For this review, take the finished solid that the model builds, in its own axes (mm). A direction names the side the tool comes from. Give positions to 0.01 mm unless a question says otherwise; leave off trailing zeros. Order: outer loops, then holes, each group sorted by start corner. A loop starts at its lowest first (then second) coordinate and runs counter-clockwise, first axis right, second up. Notation, with made-up numbers: (70, 63.5) - (110, 63.5) arc R10 ccw to (110, 76.5) - close; hole circle Ø7 at (-2, 32). An arc over 180 degrees is marked (long way). Answer as a JSON object with one key per item and string values. Group by question number.
Autodesk Inventor part; units mm, degrees
ref_plane "YZ Plane" through (0, 0, 0) normal (1, 0, 0) x (0, 1, 0)
ref_plane "XZ Plane" through (0, 0, 0) normal (0, 1, 0) x (-1, 0, 0)
ref_plane "XY Plane" through (0, 0, 0) normal (0, 0, 1) x (1, 0, 0)
sketch "Sketch1" plane through (0, 0, 0) normal (0, 0, 1) x (1, 0, 0)
  circle A0 centre (0, 0) radius 14.31
  line L0 (-76.3322, -50.4809) -> (-44.9013, -19.05)
  line L1 (0, -91.3278) -> (0, 37.4463)
  line L2 (0, -19.05) -> (-53.8815, -72.9315)
  line L3 (-53.8815, -72.9315) -> (-76.3322, -50.4809)
  line L4 (0, 19.05) -> (-105.5841, 19.05)
  line L5 (-105.5841, 19.05) -> (-159.4656, -34.8315)
  line L6 (-159.4656, -34.8315) -> (-137.015, -57.2822)
  line L7 (-137.015, -57.2822) -> (-98.7828, -19.05)
  line L8 (-98.7828, -19.05) -> (-44.9013, -19.05)
  line L9 (76.3322, -50.4809) -> (44.9013, -19.05)
  line L10 (0, -19.05) -> (53.8815, -72.9315)
  line L11 (53.8815, -72.9315) -> (76.3322, -50.4809)
  line L12 (0, 19.05) -> (105.5841, 19.05)
  line L13 (105.5841, 19.05) -> (159.4656, -34.8315)
  line L14 (159.4656, -34.8315) -> (137.015, -57.2822)
  line L15 (137.015, -57.2822) -> (98.7828, -19.05)
  line L16 (98.7828, -19.05) -> (44.9013, -19.05)
  line L17 (0, -19.05) -> (-10.6721, -29.7221)
  point P0 (-66.8959, -41.0446)
  dimension "d1" = 28.62
  dimension "d4" = 76.2
  dimension "d6" = 45
  dimension "d15" = 31.75
  dimension "d59" = 31.75
  dimension "d61" = 101.6
  dimension "d62" = 38.1
  dimension "d63" = 19.05
  dimension "d83" = 19.05
extrude "Extrusion1" add sketch "Sketch1" along normal blind 3.175 contours A0 L1 L12 L13 L14 L15 L16 L9 L11 L10 | A0 L1 L2 L3 L0 L8 L7 L6 L5 L4
sketch "Sketch3" plane through (0, 0, 3.175) normal (0, 0, 1) x (1, 0, 0)
  line L0 (53.8815, -72.9315) -> (76.3322, -50.4809)
  line L1 (76.3322, -50.4809) -> (44.9013, -19.05)
  line L2 (44.9013, -19.05) -> (98.7828, -19.05)
  line L3 (98.7828, -19.05) -> (137.015, -57.2822)
  line L4 (137.015, -57.2822) -> (159.4656, -34.8315)
  line L5 (159.4656, -34.8315) -> (105.5841, 19.05)
  line L6 (105.5841, 19.05) -> (-105.5841, 19.05)
  line L7 (-105.5841, 19.05) -> (-159.4656, -34.8315)
  line L8 (-159.4656, -34.8315) -> (-137.015, -57.2822)
  line L9 (-137.015, -57.2822) -> (-98.7828, -19.05)
  line L10 (-98.7828, -19.05) -> (-44.9013, -19.05)
  line L11 (-44.9013, -19.05) -> (-76.3322, -50.4809)
  line L12 (-76.3322, -50.4809) -> (-53.8815, -72.9315)
  line L13 (-53.8815, -72.9315) -> (0, -19.05)
  line L14 (0, -19.05) -> (53.8815, -72.9315)
  circle A0 centre (0, 0) radius 14.31
  line L15 (-148.2403, -46.0569) -> (-83.1335, 19.05)
  line L16 (-65.1069, -61.7062) -> (15.6494, 19.05)
  circle A1 centre (-139.2601, -37.0766) radius 2.65
  circle A2 centre (-121.2995, -19.1161) radius 2.65
  circle A3 centre (-103.339, -1.1556) radius 2.65
  circle A4 centre (-56.1266, -52.726) radius 2.65
  circle A5 centre (-38.1661, -34.7654) radius 2.65
  circle A6 centre (-20.2056, -16.8049) radius 2.65
  dimension "d64" = 5.3
  dimension "d67" = 25.4
  dimension "d72" = 12.7
  dimension "d73" = 12.7
  dimension "d76" = 25.4
extrude "Extrusion3" cut sketch "Sketch3" against normal blind 25.4 contours A4 L16 | L16 A4 | A5 L16 | L16 A5 | A6 L16 | L16 A6 | A3 L15 | L15 A3 | A1 L15 | L15 A1 | A2 L15 | L15 A2
mirror "Mirror2" about plane through (0, 0, 0) normal (1, 0, 0) of "Extrusion3"
fillet "Fillet1" radius 12.7 3 edges at (-98.7828, -19.05, 1.5875) (0, -19.05, 1.5875) (98.7828, -19.05, 1.5875)
fillet "Fillet2" radius 3.175 2 edges at (-44.9013, -19.05, 1.5875) (44.9013, -19.05, 1.5875)
equation "\"d1\" = bearingDiameter"
equation "\"d4\" = boltedLength"
equation "\"d6\" = 0.5 * theta12"
equation "\"d59\" = d15"
equation "\"d61\" = gearboxLength"
equation "\"topDiameter\" = 45"
equation "\"bearingDiameter\" = 28.62"
equation "\"plateThickness\" = 6.35"
equation "\"theta12\" = 90deg"
equation "\"gearboxLength\" = 101.6"
equation "\"boltedLength\" = 76.2"
equation "\"topDiameter_1\" = 25"
equation "\"shaftLength_1\" = 76.2"
equation "\"bearingDiameter_1\" = 28.62"
equation "\"plateThickness_1\" = 6.35"
equation "\"theta12_1\" = 100deg"
equation "\"boltDiameter_1\" = 6"
equation "\"gearboxLength_1\" = 101.6"
equation "\"boltedLength_1\" = 76.2"
equation "\"innerBoltSpacing_1\" = 12.7"
equation "\"outerBoltSpacing_1\" = 12.7"
equation "\"shaftLength\" = 76.2"
equation "\"boltDiameter\" = 5.3"
equation "\"outerBoltSpacing\" = 12.7"
equation "\"innerBoltSpacing\" = 12.7"
properties part number "CH1-01-KneePivotPlate" material "Aluminum 6061"
1) Consider section B-B (y = -45). Give the boundary of the cut face in (x, z) (3 decimals).
2) For faces 5 (the face through (-63.51, -37.66, 1.57)), 6 (the face through (31.12, -50.17, 1.57)), 7 (the face through (148.397, -45.9, 1.565)), list the 3-axis set-ups (+Z, -Z, +X, -X, +Y, -Y) from which the entire face can be reached by the end or side of a thin tool; tool diameter is ignored.
3) Consider section A-A (x = 0). Give the boundary of the cut face in (y, z) (3 decimals), plus the area to 3 significant figures.
4) For pin 1 (1 mm diameter, centred on x = 54, z = 2, fed in from -Y); pin 2 (1 mm diameter, centred on x = 72.5, z = 2, fed in from -Y), all flat-tipped, find the tip position at first contact; note any pin that passes through.
5) Consider section D-D (z = 1.75). Give the number of separate pieces and of enclosed holes in the cut face, plus the area to 3 significant figures.
6) Mouldability with a two-part tool opening along X and no side actions: class faces 1 (the face through (120, -40.27, 1.57)), 2 (the face through (-2, -16, 3.175)), 3 (the face through (-58.774, -52.609, 1.61)), 4 (the face through (-148.397, -45.9, 1.565)) as released by +X, released by -X, zero draft, split by the parting line, or undercut.
7) Consider section C-C (y = -60). Give the boundary of the cut face in (x, z) (3 decimals).
8) For line 1 (X direction, y = -3, z = 2.05); line 2 (X direction, y = -40, z = 1.4); line 3 (X direction, y = -18, z = 2.15), list the stretches that pass through material, from the lowest coordinate up.
Result set:
{
 "1": {"outline": "(-149.297, 0) - (-124.733, 0) - (-124.733, 3.175) - (-149.297, 3.175) - close; (-70.851, 0) - (-25.95, 0) - (-25.95, 3.175) - (-70.851, 3.175) - close; (25.95, 0) - (70.851, 0) - (70.851, 3.175) - (25.95, 3.175) - close; (124.733, 0) - (149.297, 0) - (149.297, 3.175) - (124.733, 3.175) - close"},
 "2": {"face 5": "+Z, -Z", "face 6": "+Z, -Z, -Y", "face 7": "+Z, -Z, +X, -Y"},
 "3": {"outline": "(-24.311, 0) - (-14.31, 0) - (-14.31, 3.175) - (-24.311, 3.175) - close; (14.31, 0) - (19.05, 0) - (19.05, 3.175) - (14.31, 3.175) - close", "area": "46.8 mm2"},
 "4": {"pin 1": "stops at y = -72.93", "pin 2": "stops at y = -54.81"},
 "5": {"separate pieces": "1", "enclosed holes": "13", "area": "14,900 mm2"},
 "6": {"face 1": "undercut", "face 2": "zero draft", "face 3": "undercut", "face 4": "released by -X"},
 "7": {"outline": "(-66.813, 0) - (-40.95, 0) - (-40.95, 3.175) - (-66.813, 3.175) - close; (40.95, 0) - (66.813, 0) - (66.813, 3.175) - (40.95, 3.175) - close"},
 "8": {"line 1": "x = -127.63 to -105.24, -101.44 to -13.99, 13.99 to 101.44, 105.24 to 127.63", "line 2": "x = -154.3 to -119.73, -65.85 to -20.95, 20.95 to 65.85, 119.73 to 154.3", "line 3": "x = -142.63 to -123.7, -118.9 to -22.57, -17.84 to 17.84, 22.57 to 118.9, 123.7 to 142.63"}
}
